Design review of the part shown in the three views and the two pictorial views. Dimensions are in mm from the part's minimum x, y and z. A direction names the side the tool comes from. Give positions to 0.01 mm unless a question says otherwise; leave off trailing zeros. Loops run counter-clockwise (first coordinate to the right, second up) from the corner with the lowest first, then second, coordinate; pieces in that order, holes last. Notation, with made-up numbers: (-14.75, 81.5) - (22.25, 81.5) arc R32 ccw to (22.25, 115.5) - close; hole circle Ø2 at (14.5, 36.5). An arc over 180 degrees is marked (long way). Answer as a JSON object with one key per item and string values.
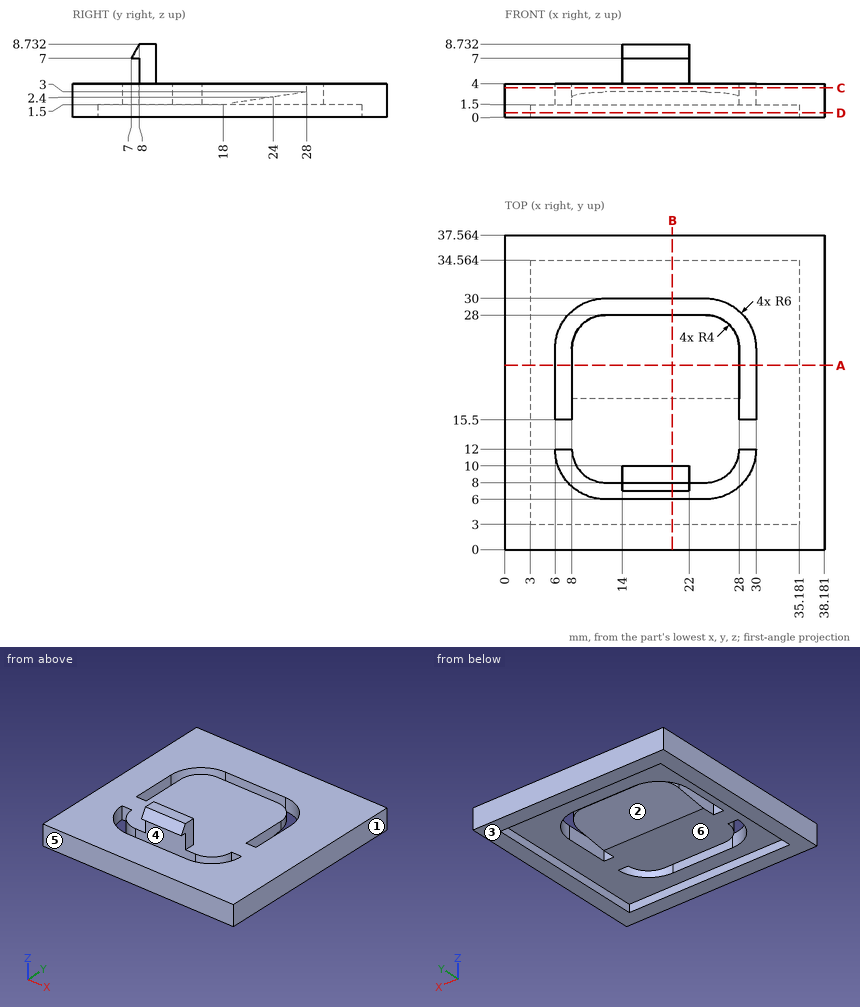
Q1. Consider section A-A, the plane y = 22. State the section outline as (x, z) points.
Results:
{"outline": "(0, 0) - (3, 0) - (3, 1.5) - (6, 1.5) - (6, 4) - (0, 4) - close; (8, 2.1) - (28, 2.1) - (28, 4) - (8, 4) - close; (30, 1.5) - (35.18, 1.5) - (35.18, 0) - (38.18, 0) - (38.18, 4) - (30, 4) - close"}
Q2. Clearance check with flat-ended pins moving along their axes: pin 1 Ø12 at (x, y) = (30, 24) entering from +Z; pin 2 Ø0.5 at (x, y) = (19, 7.5) entering from -Z; pin 3 Ø1.5 at (x, y) = (11, 33) entering from -Z. State where each tip first meets the part, or that it passes through.
Results:
{"pin 1": "stops at z = 4", "pin 2": "stops at z = 7", "pin 3": "stops at z = 1.5"}
Q3. The part is to be moulded in two halves that separate along X. For the marked faces 1, 2, 3 and 4, say which applies: +X half, -X half, draft (parallel to the pull), parting line (faces both ways), or undercut.
Results:
{"face 1": "+X half", "face 2": "undercut", "face 3": "draft", "face 4": "undercut"}
Q4. Consider section C-C, the plane z = 3.5. State the section outline as (x, y) points, plus the area to 3 significant figures.
Results:
{"outline": "(0, 0) - (38.18, 0) - (38.18, 37.56) - (0, 37.56) - close; hole (6, 12) arc R6 ccw to (12, 6) - (24, 6) arc R6 ccw to (30, 12) - (28, 12) arc R4 cw to (24, 8) - (12, 8) arc R4 cw to (8, 12) - close; hole (6, 15.5) - (8, 15.5) - (8, 24) arc R4 cw to (12, 28) - (24, 28) arc R4 cw to (28, 24) - (28, 15.5) - (30, 15.5) - (30, 24) arc R6 ccw to (24, 30) - (12, 30) arc R6 ccw to (6, 24) - close", "area": "1,290 mm^2"}
Q5. For the marked faces 5 and 6, list the 3-axis set-ups (+Z, -Z, +X, -X, +Y, -Y) from which the entire face can be reached by the end or side of a thin tool; tool diameter is ignored.
Results:
{"face 5": "+Z, -Z, +X, -X, -Y", "face 6": "-Z"}
Q6. Consider section B-B, the plane x = 20. State the section outline as (y, z) points.
Results:
{"outline": "(0, 0) - (3, 0) - (3, 1.5) - (6, 1.5) - (6, 4) - (0, 4) - close; (7, 7) - (8, 7) - (8, 1.5) - (18, 1.5) - (28, 3) - (28, 4) - (10, 4) - (10, 8.73) - (8, 8.73) - close; (30, 1.5) - (34.56, 1.5) - (34.56, 0) - (37.56, 0) - (37.56, 4) - (30, 4) - close"}
Q7. To check wall thickness, follow probe 1 along Y at (x, z) = (18, 3.5); probe 2 along Z at (x, y) = (19.5, 13.5); probe 3 along Y at (x, z) = (17, 6.25). State the ranges of each line that lie inside material, in increasing order. Write a range as [from, to].
Results:
{"probe 1": "y = [0, 6], [8, 28], [30, 37.56]", "probe 2": "z = [1.5, 4]", "probe 3": "y = [8, 10]"}
Q8. Consider section D-D, the plane z = 0.5. State the section outline as (x, y) points.
Results:
{"outline": "(0, 0) - (38.18, 0) - (38.18, 37.56) - (0, 37.56) - close; hole (3, 3) - (35.18, 3) - (35.18, 34.56) - (3, 34.56) - close"}
